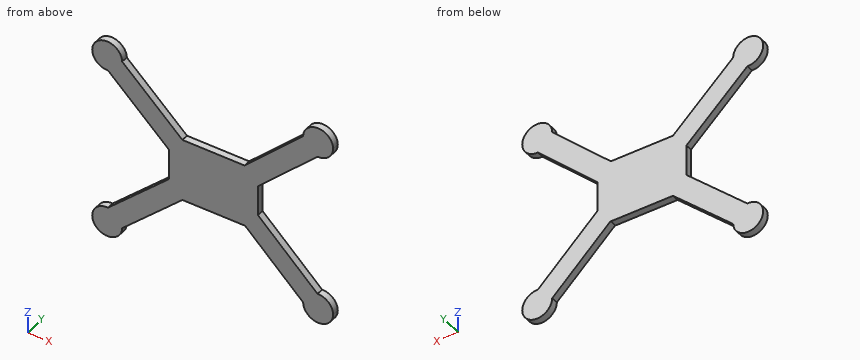
```python
from build123d import *

# Parameters (mm, degrees)
F1_DEPTH = 3.048


with BuildPart() as f1:
    # F0 (on Front) → F1 (new body)
    with BuildSketch(Plane.XZ):
        with BuildLine():
            ThreePointArc((-40.039819, 24.568676), (-40.04023, 24.642439), (-40.041462, 24.716192))
            ThreePointArc((-40.041462, 24.716192), (-51.523489, 29.074453), (-46.315227, 17.95216))
            ThreePointArc((-46.315227, 17.95216), (-41.858186, 20.009098), (-40.039819, 24.568676))
        make_face()
        with BuildLine():
            Line((-19.331162, -7.077152), (-13.392727, 0))
            Line((-13.392727, 0), (-40.041462, 24.716192))
            ThreePointArc((-40.041462, 24.716192), (-40.04023, 24.642439), (-40.039819, 24.568676))
            ThreePointArc((-40.039819, 24.568676), (-41.858186, 20.009098), (-46.315227, 17.95216))
            Line((-46.315227, 17.95216), (-19.331162, -7.077152))
        make_face()
        Polygon((14.085453, 0), (-13.392727, 0), (-19.331162, -7.077152), (-19.331162, -20.666365), (-13.392727, -27.743516), (14.085453, -27.743516), (14.209385, -27.59582), (20.023889, -20.666365), (20.023889, -20.401029), (20.023889, -7.077152), align=None)
        with BuildLine():
            Line((40.040169, 24.6367), (14.085453, 0))
            Line((14.085453, 0), (20.023889, -7.077152))
            Line((20.023889, -7.077152), (46.388558, 17.948684))
            ThreePointArc((46.388558, 17.948684), (41.86004, 20.007143), (40.040169, 24.6367))
        make_face()
        with BuildLine():
            ThreePointArc((53.291393, 24.568676), (46.699619, 31.194376), (40.040169, 24.6367))
            ThreePointArc((40.040169, 24.6367), (41.86004, 20.007143), (46.388558, 17.948684))
            ThreePointArc((46.388558, 17.948684), (51.251748, 19.786589), (53.291393, 24.568676))
        make_face()
        with BuildLine():
            Line((46.388558, -45.426865), (20.023889, -20.401029))
            Line((20.023889, -20.401029), (20.023889, -20.666365))
            Line((20.023889, -20.666365), (14.209385, -27.59582))
            Line((14.209385, -27.59582), (40.040169, -52.114881))
            ThreePointArc((40.040169, -52.114881), (41.86004, -47.485324), (46.388558, -45.426865))
        make_face()
        with BuildLine():
            ThreePointArc((53.291393, -52.046857), (51.251748, -47.26477), (46.388558, -45.426865))
            ThreePointArc((46.388558, -45.426865), (41.86004, -47.485324), (40.040169, -52.114881))
            ThreePointArc((40.040169, -52.114881), (46.699619, -58.672556), (53.291393, -52.046857))
        make_face()
        with BuildLine():
            Line((-13.392727, -27.743516), (-19.331162, -20.666365))
            Line((-19.331162, -20.666365), (-46.284951, -45.432014))
            ThreePointArc((-46.284951, -45.432014), (-41.847765, -47.498291), (-40.039819, -52.046857))
            ThreePointArc((-40.039819, -52.046857), (-40.04043, -52.13678), (-40.04226, -52.226687))
            Line((-40.04226, -52.226687), (-13.392727, -27.743516))
        make_face()
        with BuildLine():
            ThreePointArc((-40.039819, -52.046857), (-41.847765, -47.498291), (-46.284951, -45.432014))
            ThreePointArc((-46.284951, -45.432014), (-51.544735, -56.529618), (-40.04226, -52.226687))
            ThreePointArc((-40.04226, -52.226687), (-40.04043, -52.13678), (-40.039819, -52.046857))
        make_face()
    extrude(amount=F1_DEPTH)


solid = f1.part
```
Input: part model. Units: mm. Frame: model coordinates. Round coordinates to 2 decimals unless told otherwise and drop trailing zeros. Loops run counter-clockwise (first coordinate to the right, second up) from the corner with the lowest first, then second, coordinate; pieces in that order, holes last.
1) Section query B-B on x = -38. Return the cut outline in (y, z).
Ans:
outline: (-3.05, -50.35) - (0, -50.35) - (0, -37.82) - (-3.05, -37.82) - close; (-3.05, 10.24) - (0, 10.24) - (0, 22.82) - (-3.05, 22.82) - close
2) Section query A-A on z = -49.5. Return the cut outline in (x, y).
Ans:
outline: (-52.78, -3.05) - (-37.07, -3.05) - (-37.07, 0) - (-52.78, 0) - close; (37.29, -3.05) - (52.78, -3.05) - (52.78, 0) - (37.29, 0) - close
3) Pin query (flat end, axial travel): pin 1 (1.5 mm diameter, centred on x = 5.5, y = -2, fed in from +Z); pin 2 (1.5 mm diameter, centred on y = -2.5, z = 8.5, fed in from +X); pin 3 (1.5 mm diameter, centred on x = -3, y = -1.5, fed in from -Z). Return the tip coordinate at first contact, or that it passes through.
Ans:
pin 1: stops at z = 0
pin 2: stops at x = 37.22
pin 3: stops at z = -27.74
4) Section query D-D on x = -4. Return the cut outline in (y, z), plus the area to 3 significant figures.
Ans:
outline: (-3.05, -27.74) - (0, -27.74) - (0, 0) - (-3.05, 0) - close
area: 84.6 mm2
5) Material intervals for line 1 (X direction, y = -1.15, z = -55); line 2 (Z direction, x = 27, y = -1.1); line 3 (X direction, y = -2.25, z = -51.5), sorted ascending.
Ans:
line 1: x = -52.6 to -40.73, 40.73 to 52.6
line 2: z = -39.74 to -27.02, -0.46 to 12.26
line 3: x = -53.27 to -39.25, 39.39 to 53.27
6) Section query C-C on y = -2.2. Return the cut outline in (x, z), plus the area to 3 significant figures.
Ans:
outline: (-46.32, 17.95) - (-19.33, -7.08) - (-19.33, -20.67) - (-46.28, -45.43) arc R6.63 ccw (long way) to (-40.04, -52.23) - (-13.39, -27.74) - (14.09, -27.74) - (14.21, -27.6) - (40.04, -52.11) arc R6.63 ccw (long way) to (46.39, -45.43) - (20.02, -20.4) - (20.02, -7.08) - (46.39, 17.95) arc R6.63 ccw to (53.29, 24.57) arc R6.63 ccw to (40.04, 24.64) - (14.09, 0) - (-13.39, 0) - (-40.04, 24.72) arc R6.63 ccw (long way) to start
area: 2,850 mm2
